Can you work these out from the model? Positions are in its coordinate system, mm. Give positions to 0.01 mm unless a question says otherwise; leave off trailing zeros. Write each loop counter-clockwise with the first axis right and the second up, starting at its lowest first coordinate (ties: lowest second). Pieces come first, ordered by that corner, then holes. Notation, with made-up numbers: (-20.5, 34) -> (4.5, 34) arc R25 ccw to (4.5, 58) -> close; hole circle Ø1 at (78, 54.5). An arc over 180 degrees is marked (long way). Answer as CSV lines item,"result". Start each with the question number.
1. I need wall thicknesses on line 1 (X direction, y = -0.5, z = 2.1); line 2 (Y direction, x = 25, z = 4.55); line 3 (X direction, y = -6.5, z = 4.2). Which ranges of each line are inside material? Lowest first, please. Write a range as [from, to].
2. If we section it at B-B on y = -0.5: Write out the boundary of the cut face in (x, z).
3. If we section it at D-D on z = 0.95: Write out the boundary of the cut face in (x, y), plus the area to 3 significant figures.
4. If we section it at A-A on y = -8.5: Write out the boundary of the cut face in (x, z), plus the area to 3 significant figures.
5. If we section it at C-C on x = 38.5: Write out the boundary of the cut face in (y, z), plus the area to 3 significant figures.
6. I'm going to push flat-ended pins straight in: P1, Ø2.5, axis at x = 0, z = 3.5, coming from the -Y side; P2, Ø1.5, axis at x = -10, z = 3.5, coming from the +Y side. Where does each tip first touch, or does it pass through?
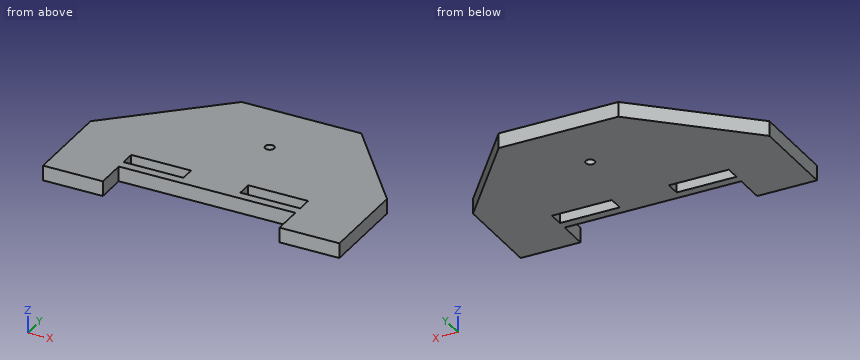
```python
from build123d import *

# Parameters (mm, degrees)
SKETCH1_R           = 1.5
SKETCH1_W           = 20
SKETCH1_H           = 4.848691284
SKETCH1_H_2         = 5
BOSS_EXTRUDE1_DEPTH = 5


with BuildPart() as part:
    # Sketch1 → Boss-Extrude1 (new body)
    with BuildSketch(Plane.XY):
        Polygon((-36.482398682, -14.486104614), (-16.482398682, -14.486104614), (-16.482398682, -4.486104614), (42.517601318, -4.486104614), (42.517601318, -14.486104614), (62.517601318, -14.486104614), (62.517601318, 15.513895386), (37.517601318, 46.513895386), (17.517601318, 46.513895386), (-2.482398682, 46.513895386), (-36.482398682, 15.513895386), align=None)
        with Locations((17.517601318, 26.513895386)):
            Circle(SKETCH1_R, mode=Mode.SUBTRACT)
        with Locations((-6.482398682, 0.938241028)):
            Rectangle(SKETCH1_W, SKETCH1_H, mode=Mode.SUBTRACT)
        with Locations((32.517601318, 1.013895386)):
            Rectangle(SKETCH1_W, SKETCH1_H_2, mode=Mode.SUBTRACT)
    extrude(amount=BOSS_EXTRUDE1_DEPTH)


solid = part.part
```
Computed values:
1,line 1,"x = [-36.48, -16.48], [3.52, 22.52], [42.52, 62.52]"
1,line 2,"y = [-4.49, -1.49], [3.51, 46.51]"
1,line 3,"x = [-36.48, -16.48], [42.52, 62.52]"
2,outline,"(-36.48, 0) -> (-16.48, 0) -> (-16.48, 5) -> (-36.48, 5) -> close; (3.52, 0) -> (22.52, 0) -> (22.52, 5) -> (3.52, 5) -> close; (42.52, 0) -> (62.52, 0) -> (62.52, 5) -> (42.52, 5) -> close"
3,outline,"(-36.48, -14.49) -> (-16.48, -14.49) -> (-16.48, -4.49) -> (42.52, -4.49) -> (42.52, -14.49) -> (62.52, -14.49) -> (62.52, 15.51) -> (37.52, 46.51) -> (-2.48, 46.51) -> (-36.48, 15.51) -> close; hole (-16.48, -1.49) -> (3.52, -1.49) -> (3.52, 3.36) -> (-16.48, 3.36) -> close; hole circle Ø3 at (17.52, 26.51); hole (22.52, -1.49) -> (42.52, -1.49) -> (42.52, 3.51) -> (22.52, 3.51) -> close"
3,area,"4,330 mm2"
4,outline,"(-36.48, 0) -> (-16.48, 0) -> (-16.48, 5) -> (-36.48, 5) -> close; (42.52, 0) -> (62.52, 0) -> (62.52, 5) -> (42.52, 5) -> close"
4,area,"200 mm2"
5,outline,"(-4.49, 0) -> (-1.49, 0) -> (-1.49, 5) -> (-4.49, 5) -> close; (3.51, 0) -> (45.3, 0) -> (45.3, 5) -> (3.51, 5) -> close"
5,area,"224 mm2"
6,P1,"stops at y = -4.49"
6,P2,"stops at y = 40.34"
